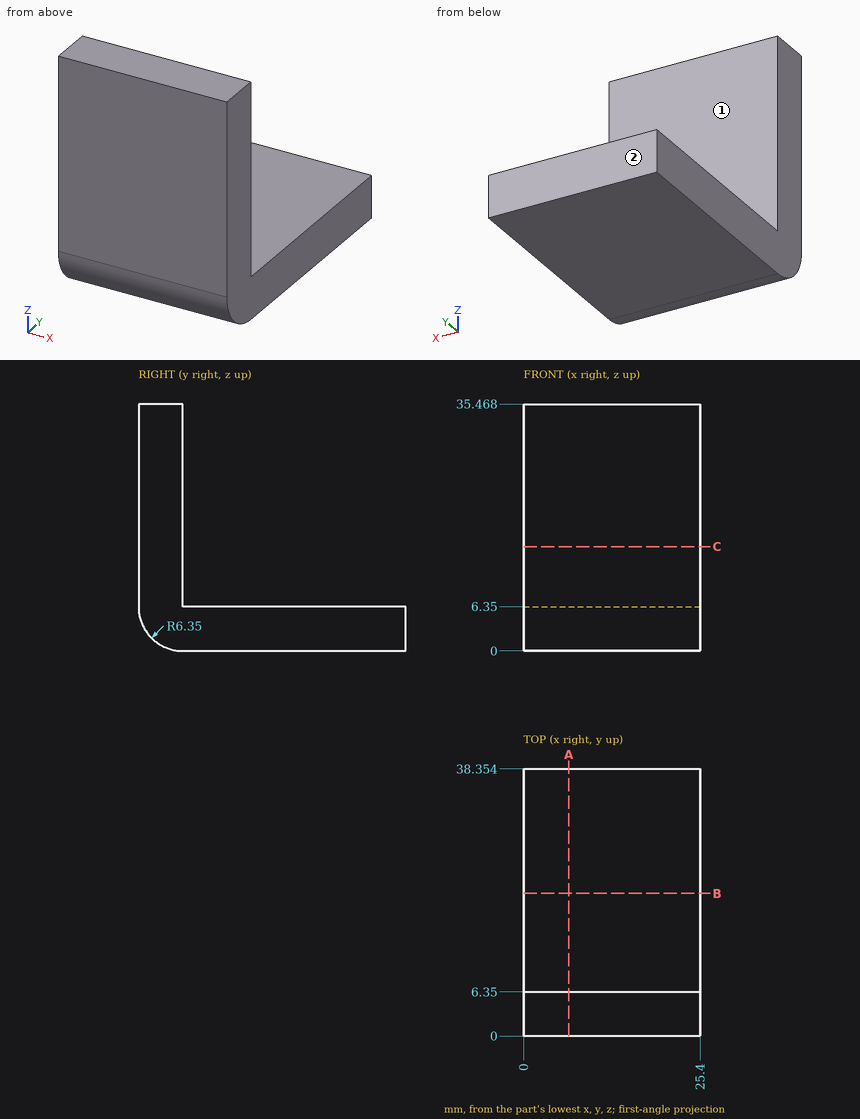
Drawing for the job (mm, zero at the part's lowest x, y, z). A direction names the side the tool comes from. Round coordinates to 2 decimals unless told otherwise and drop trailing zeros. Order: outer loops, then holes, each group sorted by start corner. A loop starts at its lowest first (then second) coordinate and runs counter-clockwise, first axis right, second up.
Item 1: Probe line 1 along Y through (x, z) = (12.75, 7); line 2 along Z through (x, y) = (14.25, 5) (1 decimal). List the from-to ranges inside material, lowest first.
Item 2: Saw through at A-A on x = 6.5. Write the cut outline in (y, z).
Item 3: Tool access for the marked faces 1 and 2: list every direction of +Z, -Z, +X, -X, +Y, -Y with a clear straight run to the whole face (end or side of a thin tool).
Item 4: Pin check, flat tips, straight feed: pin 1 (12.5 mm diameter, centred on x = 7, y = 29.5, fed in from +Z); pin 2 (7.5 mm diameter, centred on x = 7.5, z = 15, fed in from +Y). Stop position of each tip, or through.
Item 5: Saw through at B-B on y = 20.5. Write the cut outline in (x, z).
Reported:
1. line 1: y = 0 to 6.35
1. line 2: z = 0.1 to 35.5
2. outline: (0, 6.35) arc R6.35 ccw to (6.35, 0) - (38.35, 0) - (38.35, 6.35) - (6.35, 6.35) - (6.35, 35.47) - (0, 35.47) - close
3. face 1: +Z, +X, -X, +Y
3. face 2: +Z, -Z, +X, -X, +Y
4. pin 1: stops at z = 6.35
4. pin 2: stops at y = 6.35
5. outline: (0, 0) - (25.4, 0) - (25.4, 6.35) - (0, 6.35) - close
